Check sheet for the modelled part. Datum: model origin and axes. Units: mm. Coordinates: 2 decimals unless noted, no trailing zeros. Order: outer loops, then holes, each group sorted by start corner. A loop starts at its lowest first (then second) coordinate and runs counter-clockwise, first axis right, second up.
from build123d import *

# Parameters (mm, degrees)
F0_R     = 1.75
F0_R_2   = 27.5
F1_DEPTH = 2


with BuildPart() as f1:
    # F0 (on Top) → F1 (new body)
    with BuildSketch(Plane.XY):
        Polygon((14.5, 37.5), (0, 37.5), (-14.5, 37.5), (-37.5, 14.5), (-37.5, -20.5), (-30.5, -27.5), (-26.5, -27.5), (-16.5, -37.5), (-16.5, -80.5), (-14.5, -82.5), (0, -82.5), (14.5, -82.5), (16.5, -80.5), (16.5, -37.5), (26.5, -27.5), (30.5, -27.5), (37.5, -20.5), (37.5, 14.5), align=None)
        with Locations((0, -72.5)):
            Circle(F0_R, mode=Mode.SUBTRACT)
        with Locations((0, -50)):
            Circle(F0_R, mode=Mode.SUBTRACT)
        Circle(F0_R_2, mode=Mode.SUBTRACT)
    extrude(amount=F1_DEPTH)


solid = f1.part
(1) Thickness scan on probe 1 along Y at (x, z) = (0, 1.1); probe 2 along Y at (x, z) = (-8, 1.9); probe 3 along X at (y, z) = (-72.5, 1.6). Record the ranges inside material, lowest first.
Filled in:
probe 1: y = -82.5 to -74.25, -70.75 to -51.75, -48.25 to -27.5, 27.5 to 37.5
probe 2: y = -82.5 to -26.31, 26.31 to 37.5
probe 3: x = -16.5 to -1.75, 1.75 to 16.5
(2) Cross-section at B-B (z = 1.1). Enter the section's corners in (x, y), and give its area (3 significant figures).
Filled in:
outline: (-37.5, -20.5) - (-30.5, -27.5) - (-26.5, -27.5) - (-16.5, -37.5) - (-16.5, -80.5) - (-14.5, -82.5) - (14.5, -82.5) - (16.5, -80.5) - (16.5, -37.5) - (26.5, -27.5) - (30.5, -27.5) - (37.5, -20.5) - (37.5, 14.5) - (14.5, 37.5) - (-14.5, 37.5) - (-37.5, 14.5) - close; hole circle Ø55 at (0, 0); hole circle Ø3.5 at (0, -72.5); hole circle Ø3.5 at (0, -50)
area: 3,810 mm2
(3) Release check for a two-part mould opening along Y. For faces 1 (the flat face through (34, -24, 1)), 2 (the cylindrical face through (-5.961, -26.846, 0.986)), 3 (the flat face through (-1, -35, 0)) record: +Y half, -Y half, draft (parallel to the pull), parting line (faces both ways), or undercut.
Filled in:
face 1: -Y half
face 2: undercut
face 3: draft
(4) Cross-section at D-D (y = 0). Enter the section's corners in (x, z).
Filled in:
outline: (-37.5, 0) - (-27.5, 0) - (-27.5, 2) - (-37.5, 2) - close; (27.5, 0) - (37.5, 0) - (37.5, 2) - (27.5, 2) - close
(5) Go/stop test with a flat-tipped pin: P1, Ø0.6, axis at x = -29, z = 1.5, coming from the -Y side. Record where the tip stops, or that it passes through.
Filled in:
P1: stops at y = -27.5
(6) Cross-section at C-C (x = 0). Enter the section's corners in (y, z), and give its area (3 significant figures).
Filled in:
outline: (-82.5, 0) - (-74.25, 0) - (-74.25, 2) - (-82.5, 2) - close; (-70.75, 0) - (-51.75, 0) - (-51.75, 2) - (-70.75, 2) - close; (-48.25, 0) - (-27.5, 0) - (-27.5, 2) - (-48.25, 2) - close; (27.5, 0) - (37.5, 0) - (37.5, 2) - (27.5, 2) - close
area: 116 mm2
(7) Cross-section at A-A (y = -72.5). Enter the section's corners in (x, z).
Filled in:
outline: (-16.5, 0) - (-1.75, 0) - (-1.75, 2) - (-16.5, 2) - close; (1.75, 0) - (16.5, 0) - (16.5, 2) - (1.75, 2) - close
